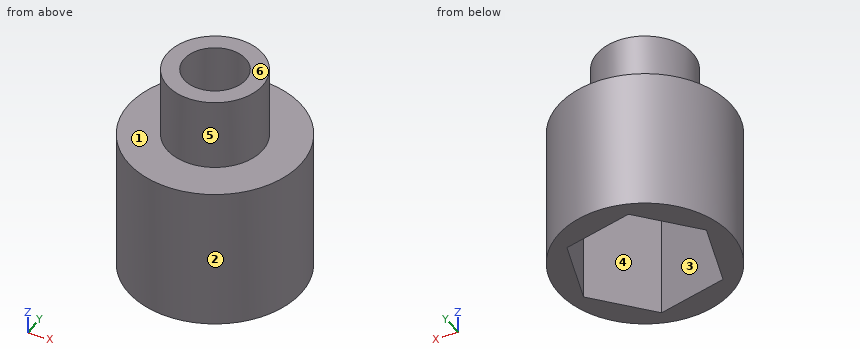
from build123d import *

# Parameters (mm, degrees)
F0_R     = 9.204375
F1_DEPTH = 12.7
F2_R     = 9.204375
F2_R_2   = 5.08
F3_DEPTH = 2.54
F2_R_3   = 3.2893
F4_DEPTH = 10.16


with BuildPart() as f1:
    # F0 (on Top) → F1 (new body)
    with BuildSketch(Plane.XY):
        with Locations((-50.731555, -47.856007)):
            Circle(F0_R)
        Polygon((-45.574418, -42.197481), (-43.252559, -49.492956), (-48.409696, -55.151481), (-55.888692, -53.514532), (-58.21055, -46.219058), (-53.053413, -40.560532), align=None, mode=Mode.SUBTRACT)
    extrude(amount=F1_DEPTH)

    # F2 (on face) → F3 (join)
    with BuildSketch(Plane.XY.offset(12.7)):
        with Locations((-50.731555, -47.856007)):
            Circle(F2_R)
        Polygon((-53.053413, -40.560532), (-45.574418, -42.197481), (-43.252559, -49.492956), (-48.409696, -55.151481), (-55.888692, -53.514532), (-58.21055, -46.219058), align=None, mode=Mode.SUBTRACT)
        Polygon((-43.252559, -49.492956), (-45.574418, -42.197481), (-53.053413, -40.560532), (-58.21055, -46.219058), (-55.888692, -53.514532), (-48.409696, -55.151481), align=None)
        with Locations((-50.731555, -47.856007)):
            Circle(F2_R_2, mode=Mode.SUBTRACT)
    extrude(amount=F3_DEPTH)

    # F2 (on face) → F4 (join)
    with BuildSketch(Plane.XY.offset(12.7)):
        with Locations((-50.731555, -47.856007)):
            Circle(F2_R_2)
        with Locations((-50.731555, -47.856007)):
            Circle(F2_R_3, mode=Mode.SUBTRACT)
    extrude(amount=F4_DEPTH)


solid = f1.part
Geometry check sheet. Reference: the model listing, model coordinates, mm. Face numbers are marked on the shaded views. A direction names the side the tool comes from. Coordinates: 2 decimals unless noted, no trailing zeros. Order: outer loops, then holes, each group sorted by start corner. A loop starts at its lowest first (then second) coordinate and runs counter-clockwise, first axis right, second up. Notation, with made-up numbers: (56.5, 57) - (87.5, 57) arc R26 cw to (87.5, 86) - close; hole circle Ø1 at (68, 49.5). An arc over 180 degrees is marked (long way). Answer in a Markdown table with one row per item. Add a question column.
1) Set-up check for the marked faces 4, 5 and 6: record each of +Z, -Z, +X, -X, +Y, -Y from which the full face is reachable in a straight line by a thin tool's end or side.
2) Cross-section at A-A, the plane y = -50.75. Record the cut outline in (x, z), then the cut area to 3 significant figures.
3) Material ranges on line 1 along Y through (x, z) = (-50.75, 11.75); line 2 along X through (y, z) = (-42.75, 2); line 3 along Y through (x, z) = (-52.75, 11.75), recorded low to high. Write a range as [from, to].
4) Cross-section at D-D, the plane x = -46. Record the cut outline in (y, z) (1 decimal).
5) Cross-section at B-B, the plane x = -50.5. Record the cut outline in (y, z).
6) Gauge pin test, flat ends, axial feed: P1, Ø5, axis at x = -47, y = -42, coming from the +Z side; P2, Ø1, axis at x = -44.5, z = 12.5, coming from the -Y side; P3, Ø4, axis at x = -47.5, y = -47.5, coming from the -Z side; P4, Ø4, axis at y = -41, z = 2.5, coming from the +X side. Record the tip position at first contact, or that the pin passes through.
7) Cross-section at C-C, the plane z = 3.25. Record the cut outline in (x, y).
8) Release check for a two-part mould opening along Y. For the marked faces 1, 2 and 3 record: +Y half, -Y half, draft (parallel to the pull), parting line (faces both ways), or undercut.
Check result:
| question | item | result |
|---|---|---|
| 1 | face 4 | -Z |
| 1 | face 5 | +Z |
| 1 | face 6 | +Z, +X, -X, +Y, -Y |
| 2 | outline | (-59.47, 0) - (-56.77, 0) - (-56.77, 12.7) - (-52.29, 12.7) - (-52.29, 22.86) - (-54.91, 22.86) - (-54.91, 15.24) - (-59.47, 15.24) - close; (-49.17, 12.7) - (-44.4, 12.7) - (-44.4, 0) - (-41.99, 0) - (-41.99, 15.24) - (-46.56, 15.24) - (-46.56, 22.86) - (-49.17, 22.86) - close |
| 2 | area | 141 mm² |
| 3 | line 1 | y = [-57.06, -54.64], [-41.06, -38.65] |
| 3 | line 2 | x = [-58.39, -55.05], [-45.4, -43.07] |
| 3 | line 3 | y = [-56.84, -54.2], [-40.63, -38.88] |
| 4 | outline | (-55.8, 0) - (-52.5, 0) - (-52.5, 12.7) - (-42.1, 12.7) - (-42.1, 0) - (-40, 0) - (-40, 15.2) - (-46, 15.2) - (-46, 22.9) - (-49.7, 22.9) - (-49.7, 15.2) - (-55.8, 15.2) - close |
| 5 | outline | (-57.06, 0) - (-54.69, 0) - (-54.69, 12.7) - (-51.14, 12.7) - (-51.14, 22.86) - (-52.93, 22.86) - (-52.93, 15.24) - (-57.06, 15.24) - close; (-44.57, 12.7) - (-41.12, 12.7) - (-41.12, 0) - (-38.65, 0) - (-38.65, 15.24) - (-42.78, 15.24) - (-42.78, 22.86) - (-44.57, 22.86) - close |
| 6 | P1 | stops at z = 22.86 |
| 6 | P2 | stops at y = -55.06 |
| 6 | P3 | stops at z = 12.7 |
| 6 | P4 | stops at x = -42.91 |
| 7 | outline | circle Ø18.41 at (-50.73, -47.86); hole (-58.21, -46.22) - (-55.89, -53.51) - (-48.41, -55.15) - (-43.25, -49.49) - (-45.57, -42.2) - (-53.05, -40.56) - close |
| 8 | face 1 | draft |
| 8 | face 2 | parting line |
| 8 | face 3 | undercut |
